Here's how the part is built. I have some questions about the finished solid (model axes, mm). A direction names the side the tool comes from. Coordinates: 2 decimals unless noted, no trailing zeros. Order: outer loops, then holes, each group sorted by start corner. A loop starts at its lowest first (then second) coordinate and runs counter-clockwise, first axis right, second up. Notation, with made-up numbers: (22, 84) - (35, 84) arc R24 ccw to (35, 101) - close; hole circle Ø5 at (-7, 65). An arc over 180 degrees is marked (long way). Use one line per item in the form item = value. Start each with the question number.
from build123d import *

# Parameters (mm, degrees)
F1_DEPTH = 7
F3_DEPTH = 50
F4_DEPTH = 100
F6_R     = 2.5
F7_DEPTH = 1.5


with BuildPart() as f1:
    # F0 (on Top) → F1 (new body)
    with BuildSketch(Plane.XY):
        with BuildLine():
            Line((5, 8), (1.5, 8))
            ThreePointArc((1.5, 8), (0, 6.5), (-1.5, 8))
            Line((-1.5, 8), (-5, 8))
            Line((-5, 8), (-5, -8))
            Line((-5, -8), (-1.5, -8))
            ThreePointArc((-1.5, -8), (0, -6.5), (1.5, -8))
            Line((1.5, -8), (5, -8))
            Line((5, -8), (5, 8))
        make_face()
        with BuildLine():
            ThreePointArc((-1.5, 8), (0, 9.5), (1.5, 8))
            Line((1.5, 8), (5, 8))
            ThreePointArc((5, 8), (0, 13), (-5, 8))
            Line((-5, 8), (-1.5, 8))
        make_face()
        with BuildLine():
            ThreePointArc((-5, -8), (0, -13), (5, -8))
            Line((5, -8), (1.5, -8))
            ThreePointArc((1.5, -8), (0, -9.5), (-1.5, -8))
            Line((-1.5, -8), (-5, -8))
        make_face()
    extrude(amount=F1_DEPTH)


with BuildPart() as f3:
    # F2 (on Front) → F3 (new body)
    with BuildSketch(Plane.XZ):
        Polygon((-3.75, 5.75), (-2.5, 7), (-5, 7), align=None)
    extrude(amount=F3_DEPTH)


with BuildPart() as f3b:
    # F2 (on Front) → F3, piece 2 (new body)
    with BuildSketch(Plane.XZ):
        Polygon((-1.25, 5.75), (0, 7), (-2.5, 7), align=None)
    extrude(amount=F3_DEPTH)


with BuildPart() as f3c:
    # F2 (on Front) → F3, piece 3 (new body)
    with BuildSketch(Plane.XZ):
        Polygon((2.5, 7), (0, 7), (1.25, 5.75), align=None)
    extrude(amount=F3_DEPTH)


with BuildPart() as f3d:
    # F2 (on Front) → F3, piece 4 (new body)
    with BuildSketch(Plane.XZ):
        Polygon((5, 7), (2.5, 7), (3.75, 5.75), align=None)
    extrude(amount=F3_DEPTH)


with BuildPart() as f4_tool:
    # F3_face (on face) → F4 (new body)
    with BuildSketch(Plane(origin=(-3.75, -50, 6.5833333333), x_dir=(1, 0, 0), z_dir=(0, -1, 0))):
        Polygon((0, -0.8333333333), (1.25, 0.4166666667), (-1.25, 0.4166666667), align=None)
        Polygon((2.5, -0.8333333333), (3.75, 0.4166666667), (1.25, 0.4166666667), align=None)
        Polygon((6.25, 0.4166666667), (3.75, 0.4166666667), (5, -0.8333333333), align=None)
        Polygon((8.75, 0.4166666667), (6.25, 0.4166666667), (7.5, -0.8333333333), align=None)
    extrude(amount=-F4_DEPTH)


with BuildPart() as f1_1:
    add(f1.part)

    # F4: cut by f4_tool
    add(f4_tool.part, mode=Mode.SUBTRACT)

    # F6 (on offset) → F7 (cut)
    with BuildSketch(Plane.XY.offset(7)):
        with Locations((0, -8)):
            Circle(F6_R)
        with Locations((0, 8)):
            Circle(F6_R)
    extrude(amount=-F7_DEPTH, mode=Mode.SUBTRACT)


with BuildPart() as f3_1:
    add(f3.part)

    # F4: cut by f4_tool
    add(f4_tool.part, mode=Mode.SUBTRACT)


with BuildPart() as f3b_1:
    add(f3b.part)

    # F4: cut by f4_tool
    add(f4_tool.part, mode=Mode.SUBTRACT)


with BuildPart() as f3c_1:
    add(f3c.part)

    # F4: cut by f4_tool
    add(f4_tool.part, mode=Mode.SUBTRACT)


with BuildPart() as f3d_1:
    add(f3d.part)

    # F4: cut by f4_tool
    add(f4_tool.part, mode=Mode.SUBTRACT)


solid = f1_1.part
1) Which directions (+Z, -Z, +X, -X, +Y, -Y) give clear straight access to the entire face, cutting with the end or side of a thin tool? Please do faces 1 (the cylindrical face through (0.325, 6.536, 2.712)), 2 (the cylindrical face through (-2.5, -7.9, 6.1)), 3 (the flat face through (3.1, -0.2, 6.4)).
2) Suppose I cut it at B-B, the plane y = -5.25. List the corners of the cut face in (x, z) for me.
3) Suppose I cut it at D-D, the plane y = 8.5. List the corners of the cut face in (x, z) for me.
4) Suppose I cut it at A-A, the plane x = -1. List the corners of the cut face in (y, z) for me, then the cut area to 3 significant figures.
5) I need wall thicknesses on probe 1 along Y at (x, z) = (0, 6.4); probe 2 along Y at (x, z) = (0, 2.7); probe 3 along X at (y, z) = (-8, 6.4). Which ranges of each line are inside material? Lowest first, please. Write a range as [from, to].
6) Suppose I cut it at C-C, the plane z = 2. List the corners of the cut face in (x, y) for me.
7) For pin 1 (2.5 mm diameter, centred on x = 0, y = 9, fed in from +Z); pin 2 (3.5 mm diameter, centred on x = 0, y = 8, fed in from -Z), each with a flat end and sliding along its axis, tell me the tip position at first contact or that it passes through.
From the geometry:
q1.face_1 = +Z, -Z
q1.face_2 = +Z
q1.face_3 = +Z, +Y, -Y
q2.outline = (-5, 0) - (5, 0) - (5, 7) - (3.75, 5.75) - (2.5, 7) - (1.25, 5.75) - (0, 7) - (-1.25, 5.75) - (-2.5, 7) - (-3.75, 5.75) - (-5, 7) - close
q3.outline = (-4.97, 0) - (-1.41, 0) - (-1.41, 5.5) - (-2.45, 5.5) - (-2.45, 6.95) - (-2.5, 7) - (-3.75, 5.75) - (-4.97, 6.97) - close; (1.41, 0) - (4.97, 0) - (4.97, 6.97) - (3.75, 5.75) - (2.5, 7) - (2.45, 6.95) - (2.45, 5.5) - (1.41, 5.5) - close
q4.outline = (-12.9, 0) - (-9.12, 0) - (-9.12, 5.5) - (-10.29, 5.5) - (-10.29, 6) - (-12.9, 6) - close; (-6.88, 0) - (6.88, 0) - (6.88, 5.5) - (5.71, 5.5) - (5.71, 6) - (-5.71, 6) - (-5.71, 5.5) - (-6.88, 5.5) - close; (9.12, 0) - (12.9, 0) - (12.9, 6) - (10.29, 6) - (10.29, 5.5) - (9.12, 5.5) - close
q4.area = 126 mm2
q5.probe_1 = [-13, -10.5], [-5.5, 5.5], [10.5, 13]
q5.probe_2 = [-13, -9.5], [-6.5, 6.5], [9.5, 13]
q5.probe_3 = [-5, -4.4], [-3.1, -2.5], [2.5, 3.1], [4.4, 5]
q6.outline = (-5, -8) arc R5 ccw to (5, -8) - (5, 8) arc R5 ccw to (-5, 8) - close; hole circle Ø3 at (0, -8); hole circle Ø3 at (0, 8)
q7.pin_1 = 5.5
q7.pin_2 = 0
